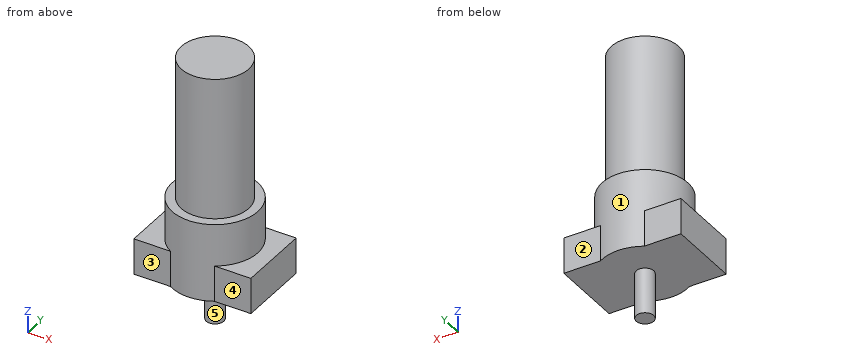
```python
from build123d import *

# Parameters (mm, degrees)
SKETCH_1_R      = 10
EXTRUDE_1_DEPTH = 51.9
SKETCH_2_R      = 48.877397639
EXTRUDE_2_DEPTH = 89
SKETCH_4_W      = 133.6
SKETCH_4_H      = 84
EXTRUDE_4_DEPTH = 41
SKETCH_5_R      = 38.5
EXTRUDE_5_DEPTH = 251


with BuildPart() as part:
    # 草图1 → 凸台-拉伸1 (new body)
    with BuildSketch(Plane.XY):
        with Locations(Location((0, 0, 0), (0, 0, 180))):
            Circle(SKETCH_1_R)
    extrude(amount=EXTRUDE_1_DEPTH)

    # 草图2 → 凸台-拉伸2 (add)
    with BuildSketch(Plane.XY.offset(51.9)):
        Circle(SKETCH_2_R)
    extrude(amount=EXTRUDE_2_DEPTH)

    # 草图4 → 凸台-拉伸4 (add)
    with BuildSketch(Plane(origin=(0, 0, 51.9), x_dir=(-1, 0, 0), z_dir=(0, 0, -1))):
        Rectangle(SKETCH_4_W, SKETCH_4_H)
    extrude(amount=-EXTRUDE_4_DEPTH)

    # 草图5 → 凸台-拉伸5 (add)
    with BuildSketch(Plane(origin=(0, 0, 51.9), x_dir=(-1, 0, 0), z_dir=(0, 0, -1))):
        Circle(SKETCH_5_R)
    extrude(amount=-EXTRUDE_5_DEPTH)


solid = part.part
```
Work out the finished part from the listing and answer in its coordinate system (mm). Face numbers are marked on the shaded views. A direction names the side the tool comes from. Round coordinates to 2 decimals unless told otherwise and drop trailing zeros. Write each loop counter-clockwise with the first axis right and the second up, starting at its lowest first coordinate (ties: lowest second). Pieces come first, ordered by that corner, then holes. Notation, with made-up numbers: (-1.75, 11.25) -> (53.25, 11.25) arc R9 ccw to (53.25, 23.25) -> close; hole circle Ø6 at (26.5, 70.25). An arc over 180 degrees is marked (long way). Write each question's results on one line, items separated by ' | '.
1) The part is cut by section C-C (z = 71). Write down the section's boundary in (x, y), and give its area (3 significant figures).
Findings:
outline: (-66.8, -42) -> (-25, -42) arc R48.88 ccw to (25, -42) -> (66.8, -42) -> (66.8, 42) -> (25, 42) arc R48.88 ccw to (-25, 42) -> (-66.8, 42) -> close | area: 11,700 mm²
2) Consider line 1 along Z through (x, y) = (31, -1.5); line 2 along Z through (x, y) = (60, 4); line 3 along Y through (x, z) = (27, 286.5). Determine where each line is inside the solid, lowest interval first. Write a range as [from, to].
Findings:
line 1: z = [51.9, 302.9] | line 2: z = [51.9, 92.9] | line 3: y = [-27.45, 27.45]
3) The part is cut by section A-A (y = 0). Write down the section's boundary in (x, z).
Findings:
outline: (-66.8, 51.9) -> (-10, 51.9) -> (-10, 0) -> (10, 0) -> (10, 51.9) -> (66.8, 51.9) -> (66.8, 92.9) -> (48.88, 92.9) -> (48.88, 140.9) -> (38.5, 140.9) -> (38.5, 302.9) -> (-38.5, 302.9) -> (-38.5, 140.9) -> (-48.88, 140.9) -> (-48.88, 92.9) -> (-66.8, 92.9) -> close
4) The part is cut by section D-D (x = -19.5). Write down the section's boundary in (y, z).
Findings:
outline: (-44.82, 51.9) -> (44.82, 51.9) -> (44.82, 140.9) -> (33.2, 140.9) -> (33.2, 302.9) -> (-33.2, 302.9) -> (-33.2, 140.9) -> (-44.82, 140.9) -> close
5) Flat-ended cylindrical pins translate along their axes: pin 1 (12.5 mm diameter, centred on x = -48.5, z = 68.5, fed in from +Y); pin 2 (12 mm diameter, centred on x = 26.5, y = 37, fed in from +Z); pin 3 (5 mm diameter, centred on y = -31, z = 270.5, fed in from -X). Find the tip coordinate at first contact, or state that the pin passes through.
Findings:
pin 1: stops at y = 42 | pin 2: stops at z = 140.9 | pin 3: stops at x = -25.88
6) Which of the six approach directions +Z, -Z, +X, -X, +Y, -Y give full straight-line access (tool end or side, diameter ignored) to the marked faces 1, 2, 3, 4 and 5?
Findings:
face 1: +Z | face 2: +Z, -Z, +X, +Y | face 3: +Z, -Z, -X, -Y | face 4: +Z, -Z, +X, -Y | face 5: -Z
7) The part is cut by section B-B (x = 0). Write down the section's boundary in (y, z), and give its area (3 significant figures).
Findings:
outline: (-48.88, 51.9) -> (-10, 51.9) -> (-10, 0) -> (10, 0) -> (10, 51.9) -> (48.88, 51.9) -> (48.88, 140.9) -> (38.5, 140.9) -> (38.5, 302.9) -> (-38.5, 302.9) -> (-38.5, 140.9) -> (-48.88, 140.9) -> close | area: 22,200 mm²
